```python
from build123d import *

# Parameters (mm, degrees)
SKETCH_1_R               = 4.5
EXTRUDE_1_DEPTH          = 3
SKETCH_2_R               = 3
EXTRUDE_2_DEPTH          = 26.2
SKETCH_6_R               = 1.5
EXTRUDE_3_DEPTH          = 1.25
SKETCH_8_OUTSIDE_W       = 18.018
SKETCH_8_OUTSIDE_H       = 18.018
SKETCH_8_OUTSIDE_R       = 3
CUT_EXTRUDE_3_DEPTH      = 31.374166655
SKETCH_4_R               = 2.75
CUT_EXTRUDE_1_DEPTH      = 22.2
FILLET_2_R               = 1
EXTRUDE_4_REACH          = 40.314
EXTRUDE_4_END_RADIUS     = 3
EXTRUDE_START            = 5
SKETCH_9_R               = 0.5
CUT_EXTRUDE_4_REACH      = 36.348
CUT_EXTRUDE_4_END_RADIUS = 2.75
SKETCH_10_R              = 0.25
FILLET_3_R               = 0.3


with BuildPart() as part:
    # 草圖1 → 填料-伸長1 (new body)
    with BuildSketch(Plane.XY):
        Circle(SKETCH_1_R)
    extrude(amount=-EXTRUDE_1_DEPTH)

    # 草圖2 → 填料-伸長2 (add)
    with BuildSketch(Plane.XY):
        Circle(SKETCH_2_R)
    extrude(amount=-EXTRUDE_2_DEPTH)

    # 草圖6 → 填料-伸長3 (add, symmetric)
    with BuildSketch(Plane(origin=(0, 0, 0), x_dir=(1, 0, 0), z_dir=(0, 1, 0))):
        with BuildLine():
            Line((-3, 26.2), (-2.482050808, 30.499038106))
            ThreePointArc((-2.482050808, 30.499038106), (0, 32.7), (2.482050808, 30.499038106))
            Line((2.482050808, 30.499038106), (3, 26.2))
            Line((3, 26.2), (-3, 26.2))
        make_face()
        with Locations(Location((0, 30.2, 0), (0, 0, 270))):
            Circle(SKETCH_6_R, mode=Mode.SUBTRACT)
    extrude(amount=EXTRUDE_3_DEPTH, both=True)

    # 草圖8 outside → 除料-伸長3 (cut, through all)
    with BuildSketch(Plane(origin=(0, 0, -3), x_dir=(-1, 0, 0), z_dir=(0, 0, -1))):
        Rectangle(SKETCH_8_OUTSIDE_W, SKETCH_8_OUTSIDE_H)
        with Locations(Location((0, 0, 0), (0, 0, 180))):
            Circle(SKETCH_8_OUTSIDE_R, mode=Mode.SUBTRACT)
    extrude(amount=CUT_EXTRUDE_3_DEPTH, mode=Mode.SUBTRACT)

    # 草圖4 → 除料-伸長1 (cut)
    with BuildSketch(Plane.XY):
        Circle(SKETCH_4_R)
    extrude(amount=-CUT_EXTRUDE_1_DEPTH, mode=Mode.SUBTRACT)

    # 圓角2
    fillet_2_edges = [part.edges().sort_by_distance(p)[0] for p in [
        (-2.75, 0, -22.2),
    ]]
    fillet(fillet_2_edges, radius=FILLET_2_R)

    # 填料-伸長4: up to this cylinder (the profile starts outside it)
    extrude_4_end = Plane(origin=(0, 0, -20), z_dir=(0, 0, 1)) * Cylinder(EXTRUDE_4_END_RADIUS, 87.628, mode=Mode.PRIVATE)
    # 草圖9 → 填料-伸長4 (add, up to the surface)
    with BuildSketch(Plane(origin=(0, 0, 0), x_dir=(1, 0, 0), z_dir=(0, 1, 0)).offset(EXTRUDE_START), mode=Mode.PRIVATE) as extrude_4_sk1:
        with Locations(Location((0, 20, 0), (0, 0, 270))):
            Circle(SKETCH_9_R)
    extrude_4_tool1 = extrude(extrude_4_sk1.sketch, amount=-EXTRUDE_4_REACH, mode=Mode.PRIVATE) - extrude_4_end
    add(extrude_4_tool1.solids().sort_by_distance((0, 5, -20))[0])

    # 除料-伸長4: up to this cylinder (the profile starts outside it)
    cut_extrude_4_end = Plane(origin=(0, 0, -20), z_dir=(0, 0, 1)) * Cylinder(CUT_EXTRUDE_4_END_RADIUS, 79.196, mode=Mode.PRIVATE)
    # 草圖10 → 除料-伸長4 (cut, up to the surface)
    with BuildSketch(Plane(origin=(0, 5, 0), x_dir=(1, 0, 0), z_dir=(0, 1, 0)), mode=Mode.PRIVATE) as cut_extrude_4_sk1:
        with Locations(Location((0, 20, 0), (0, 0, 270))):
            Circle(SKETCH_10_R)
    cut_extrude_4_tool1 = extrude(cut_extrude_4_sk1.sketch, amount=-CUT_EXTRUDE_4_REACH, mode=Mode.PRIVATE) - cut_extrude_4_end
    add(cut_extrude_4_tool1.solids().sort_by_distance((0, 5, -20))[0], mode=Mode.SUBTRACT)

    # 圓角3
    fillet_3_edges = [part.edges().sort_by_distance(p)[0] for p in [
        (0, 3, -20.5),
    ]]
    fillet(fillet_3_edges, radius=FILLET_3_R)


solid = part.part
```
Read the model definition and answer for the solid it produces. Units are mm, in the model's axes. A direction names the side the tool comes from. Give positions to 0.01 mm unless a question says otherwise; leave off trailing zeros. Write each loop counter-clockwise with the first axis right and the second up, starting at its lowest first coordinate (ties: lowest second). Pieces come first, ordered by that corner, then holes. Notation, with made-up numbers: (-17, 12) -> (19, 12) arc R23 ccw to (19, 30) -> close; hole circle Ø8 at (-25, -9). An arc over 180 degrees is marked (long way). Answer as a JSON object with one key per item and string values.
1) Section D-D on z = -24.5 is taken. Write down the section's boundary in (x, y).
Findings below:
{"outline": "circle Ø6 at (0, 0)"}
2) Section A-A on y = 0 is taken. Write down the section's boundary in (x, z).
Findings below:
{"outline": "(-4.5, -3) -> (-3, -3) -> (-3, -26.2) -> (-2.48, -30.5) arc R2.5 ccw to (2.48, -30.5) -> (3, -26.2) -> (3, -3) -> (4.5, -3) -> (4.5, 0) -> (2.75, 0) -> (2.75, -21.2) arc R1 cw to (1.75, -22.2) -> (-1.75, -22.2) arc R1 cw to (-2.75, -21.2) -> (-2.75, 0) -> (-4.5, 0) -> close; hole circle Ø3 at (0, -30.2)"}
3) A tool of negligible diameter and unlimited length cuts with its end or side. For faces 5 (the cylindrical face through (-0.596, -2.685, -10.452)), 6 (the flat face through (0, 2, -26.2)), 7 (the cylindrical face through (0.15, 4.113, -19.523)), 8 (the flat face through (0, -2, -26.2)), from which of +Z, -Z, +X, -X, +Y, -Y can it reach the whole face along a straight path? Write none if from no direction.
Findings below:
{"face 5": "+Z", "face 6": "-Z, +X, -X, +Y", "face 7": "+Y", "face 8": "-Z, +X, -X, -Y"}
4) Straight lines are drawn through the part: probe 1 along Z at (x, y) = (0, 3.35); probe 2 along X at (y, z) = (4.1, -20); probe 3 along Z at (x, y) = (-1.75, 2.25). For each, find the intervals that lie inside material, in ascending order. Write a range as from..to.
Findings below:
{"probe 1": "z = -20.5..-20.25, -19.75..-19.5, -3..0", "probe 2": "x = -0.5..-0.25, 0.25..0.5", "probe 3": "z = -26.2..0"}
5) Section B-B on z = -30.2 is taken. Write down the section's boundary in (x, y), then the cut area to 3 significant figures.
Findings below:
{"outline": "(-2.52, -1.25) -> (-1.5, -1.25) -> (-1.5, 1.25) -> (-2.52, 1.25) -> close; (1.5, -1.25) -> (2.52, -1.25) -> (2.52, 1.25) -> (1.5, 1.25) -> close", "area": "5.09 mm^2"}
6) For a pull along Y with two mould halves and no side action, classify faces 1 (the cylindrical face through (0.45, -0.02, -28.77)), 2 (the flat face through (0, -1.25, -28)), 3 (the flat face through (0, 1.25, -28)), 4 (the flat face through (0, 0, -22.2)) as pulls with the +Y half, pulls with the -Y half, needs draft (parallel to the pull), parting line crosses it, or undercut.
Findings below:
{"face 1": "needs draft", "face 2": "pulls with the -Y half", "face 3": "pulls with the +Y half", "face 4": "undercut"}
7) Section C-C on z = -6 is taken. Write down the section's boundary in (x, y), then the cut area to 3 significant figures.
Findings below:
{"outline": "circle Ø6 at (0, 0); hole circle Ø5.5 at (0, 0)", "area": "4.52 mm^2"}
8) Flat-ended cylindrical pins translate along their axes: pin 1 Ø1.9 at (x, y) = (-1, 2) entering from -Z (3 decimals); pin 2 Ø2 at (x, z) = (-1.5, -22.5) entering from +Y; pin 3 Ø1.6 at (x, z) = (-0.5, -31) entering from -Y. Find the tip coordinate at first contact, or state that the pin passes through.
Findings below:
{"pin 1": "stops at z = -32.665", "pin 2": "stops at y = 2.96", "pin 3": "stops at y = -1.25"}
